Verification items for this drawing (mm, ordinates from the low corner). A direction names the side the tool comes from. Coordinates: 2 decimals unless noted, no trailing zeros. Write each loop counter-clockwise with the first axis right and the second up, starting at its lowest first coordinate (ties: lowest second). Pieces come first, ordered by that corner, then holes. Notation, with made-up numbers: (16.25, 88.5) -> (37.25, 88.5) arc R17 cw to (37.25, 101.5) -> close; hole circle Ø3 at (22, 77). An arc over 180 degrees is marked (long way). Put each result on its own line as item: value. Start each with the question number.
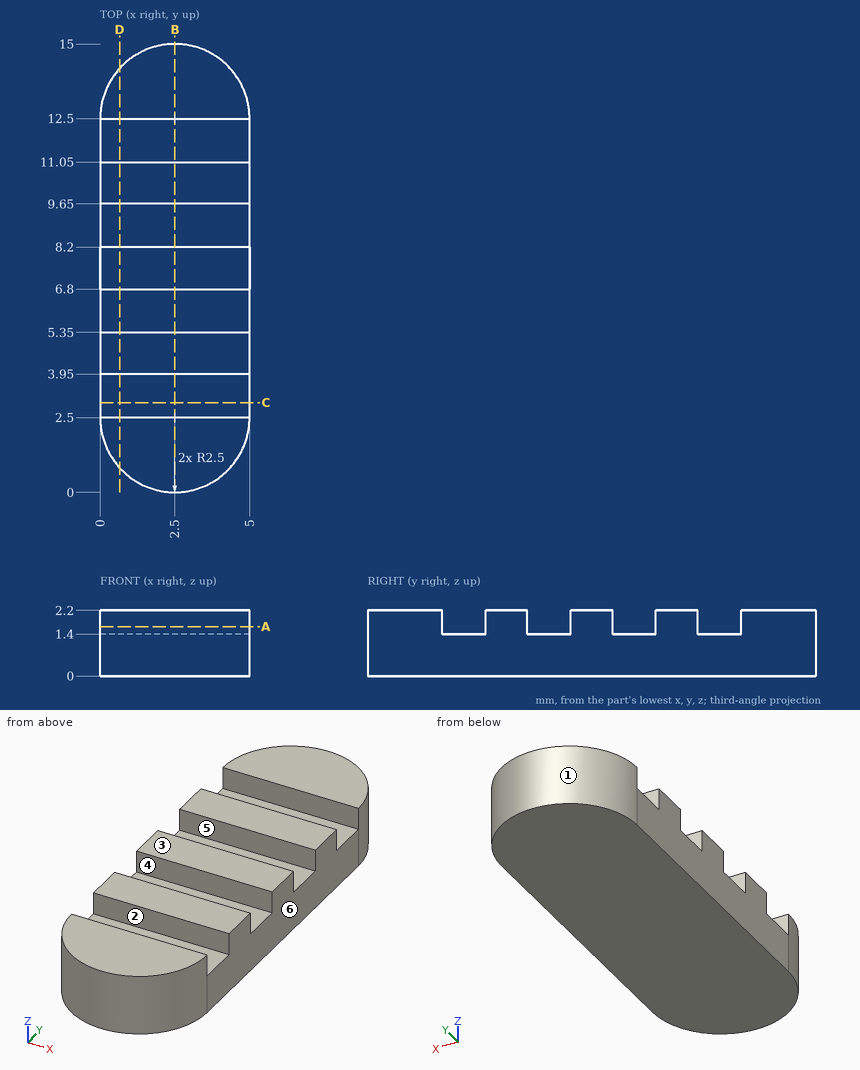
Item 1: Access from +Z, -Z, +X, -X, +Y, -Y to the whole of each face (thin tool, end or side, straight path). Record for the marked faces 5 and 6.
Item 2: Mould release check, pull along Y, two halves, no side actions. Record for the marked faces 1, 2, 3 and 4: released by +Y, released by -Y, zero draft, split by the parting line, or undercut.
Item 3: Section check D-D, the plane x = 0.65. Enter the section's corners in (y, z).
Item 4: Section check C-C, the plane y = 3. Enter the section's corners in (x, z).
Item 5: Scan lines: line 1 along Y through (x, z) = (3.05, 1.8); line 2 along Y through (x, z) = (0.85, 1.5); line 3 along Z through (x, y) = (2.9, 5.75). Record each from-to range of solid material in increasing order. Write a range as [from, to].
Item 6: Section check A-A, the plane z = 1.65. Enter the section's corners in (x, y).
Item 7: Go/stop test with flat-tipped pins: P1, Ø0.9, axis at x = 3.5, z = 1.5, coming from the +Y side; P2, Ø1.2, axis at x = 3.5, y = 9, coming from the +Z side; P3, Ø0.6, axis at x = 3.5, z = 1.5, coming from the -Y side. Record where each tip stops, or that it passes through.
Item 8: Section check B-B, the plane x = 2.5. Enter the section's corners in (y, z).
From the geometry:
1. face 5: +Z, +X, -X
1. face 6: +Z, -Z, +X, +Y, -Y
2. face 1: released by +Y
2. face 2: undercut
2. face 3: zero draft
2. face 4: undercut
3. outline: (0.82, 0) -> (14.18, 0) -> (14.18, 2.2) -> (12.5, 2.2) -> (12.5, 1.4) -> (11.05, 1.4) -> (11.05, 2.2) -> (9.65, 2.2) -> (9.65, 1.4) -> (8.2, 1.4) -> (8.2, 2.2) -> (6.8, 2.2) -> (6.8, 1.4) -> (5.35, 1.4) -> (5.35, 2.2) -> (3.95, 2.2) -> (3.95, 1.4) -> (2.5, 1.4) -> (2.5, 2.2) -> (0.82, 2.2) -> close
4. outline: (0, 0) -> (5, 0) -> (5, 1.4) -> (0, 1.4) -> close
5. line 1: [0.06, 2.5], [3.95, 5.35], [6.8, 8.2], [9.65, 11.05], [12.5, 14.94]
5. line 2: [0.62, 2.5], [3.95, 5.35], [6.8, 8.2], [9.65, 11.05], [12.5, 14.38]
5. line 3: [0, 1.4]
6. outline: (0, 2.5) arc R2.5 ccw to (5, 2.5) -> close; (0, 3.95) -> (5, 3.95) -> (5, 5.35) -> (0, 5.35) -> close; (0, 6.8) -> (5, 6.8) -> (5, 8.2) -> (0, 8.2) -> close; (0, 9.65) -> (5, 9.65) -> (5, 11.05) -> (0, 11.05) -> close; (0, 12.5) -> (5, 12.5) arc R2.5 ccw to start
7. P1: y = 14.94
7. P2: z = 1.4
7. P3: y = 0.1
8. outline: (0, 0) -> (15, 0) -> (15, 2.2) -> (12.5, 2.2) -> (12.5, 1.4) -> (11.05, 1.4) -> (11.05, 2.2) -> (9.65, 2.2) -> (9.65, 1.4) -> (8.2, 1.4) -> (8.2, 2.2) -> (6.8, 2.2) -> (6.8, 1.4) -> (5.35, 1.4) -> (5.35, 2.2) -> (3.95, 2.2) -> (3.95, 1.4) -> (2.5, 1.4) -> (2.5, 2.2) -> (0, 2.2) -> close
